```python
from build123d import *

# Parameters (mm, degrees)
SKETCH1_W      = 200
SKETCH1_H      = 155
SKETCH1_W_2    = 191
SKETCH1_H_2    = 146
SKETCH1_W_3    = 5
SKETCH1_H_3    = 2.5
SKETCH1_W_4    = 2.5
SKETCH1_H_4    = 5
MAINBODY_DEPTH = 20


with BuildPart() as part:
    # Sketch1 → MainBody (new body)
    with BuildSketch(Plane(origin=(0, 0, 0), x_dir=(1, 0, 0), z_dir=(0, 1, 0))):
        Rectangle(SKETCH1_W, SKETCH1_H)
        Rectangle(SKETCH1_W_2, SKETCH1_H_2, mode=Mode.SUBTRACT)
        with Locations((93.5, -75.25)):
            Rectangle(SKETCH1_W_3, SKETCH1_H_3, mode=Mode.SUBTRACT)
        with Locations((-93.5, -75.25)):
            Rectangle(SKETCH1_W_3, SKETCH1_H_3, mode=Mode.SUBTRACT)
        with Locations((97.75, -20)):
            Rectangle(SKETCH1_W_4, SKETCH1_H_4, mode=Mode.SUBTRACT)
        with Locations((97.75, 74)):
            Rectangle(SKETCH1_W_4, SKETCH1_H_4, mode=Mode.SUBTRACT)
        with Locations((-97.75, -20)):
            Rectangle(SKETCH1_W_4, SKETCH1_H_4, mode=Mode.SUBTRACT)
        with Locations((-97.75, 74)):
            Rectangle(SKETCH1_W_4, SKETCH1_H_4, mode=Mode.SUBTRACT)
    extrude(amount=MAINBODY_DEPTH)


solid = part.part
```
Part model, mm, in its own coordinate system. A direction names the side the tool comes from. Give positions to 0.01 mm unless a question says otherwise; leave off trailing zeros. Order: outer loops, then holes, each group sorted by start corner. A loop starts at its lowest first (then second) coordinate and runs counter-clockwise, first axis right, second up. Notation, with made-up numbers: (87, 31) - (103, 31) arc R28 ccw to (103, 51) - close; hole circle Ø10 at (73, -19). An arc over 180 degrees is marked (long way). Use one line per item in the form item = value.
Item 1: Slice it at A-A on x = 53. Give the cut face in (y, z), and give its area (3 significant figures).
Solution:
outline = (0, -77.5) - (20, -77.5) - (20, -73) - (0, -73) - close; (0, 73) - (20, 73) - (20, 77.5) - (0, 77.5) - close
area = 180 mm2
Item 2: Which spindle directions (+Z, -Z, +X, -X, +Y, -Y) get a long thin tool onto all of the face, cutting with end or side? Do faces 1 (the face through (99, 10, 20)), 2 (the face through (-1, 10, -77.5)). Say none if no direction does.
Solution:
face_1 = +Y, -Y
face_2 = -Z, +X, -X, +Y, -Y
Item 3: Slice it at C-C on y = 9.5. Count the separate pieces of the cut face and the enclosed holes in it, and give its area (3 significant figures).
Solution:
separate_pieces = 1
enclosed_holes = 7
area = 3,040 mm2
Item 4: Probe probe 1 along X at (y, z) = (9, 18.5); probe 2 along X at (y, z) = (16.5, -42); probe 3 along Z at (x, y) = (-89, 4.75). List the from-to ranges inside material, lowest first. Write a range as from..to.
Solution:
probe_1 = -100..-99, -96.5..-95.5, 95.5..96.5, 99..100
probe_2 = -100..-95.5, 95.5..100
probe_3 = -77.5..-73, 73..77.5
Item 5: Slice it at B-B on z = 41.5. Give the cut face in (x, y), and give its area (3 significant figures).
Solution:
outline = (-100, 0) - (-95.5, 0) - (-95.5, 20) - (-100, 20) - close; (95.5, 0) - (100, 0) - (100, 20) - (95.5, 20) - close
area = 180 mm2
Item 6: Two-plate mould, pull along X, no slides. Class faces 3 (the face through (100, 10, 1)), 4 (the face through (-8, 0, 74)), 5 (the face through (93, 10, 76.5)): released by +X, released by -X, zero draft, split by the parting line, or undercut.
Solution:
face_3 = released by +X
face_4 = zero draft
face_5 = undercut
